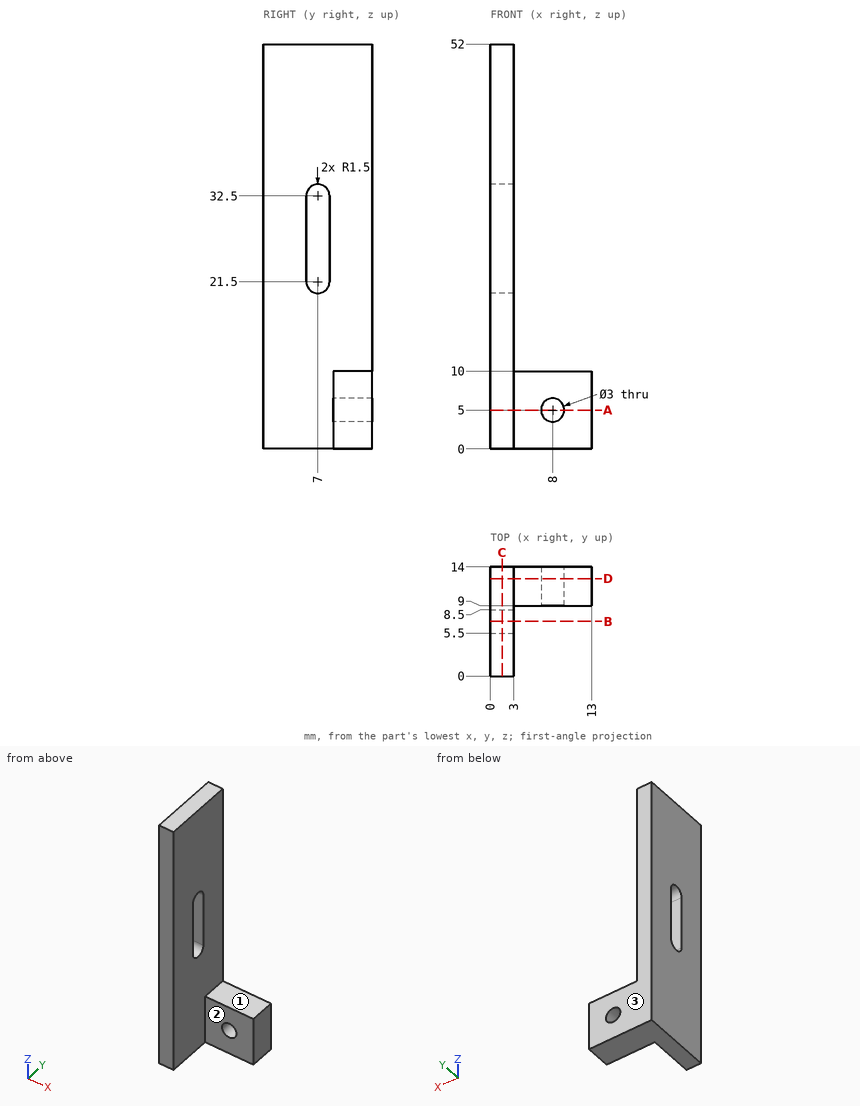
Job drawing, mm, ordinate dimensions from the low corner. One solid piece. Give positions to 0.01 mm unless a question says otherwise; leave off trailing zeros. Loops run counter-clockwise (first coordinate to the right, second up) from the corner with the lowest first, then second, coordinate; pieces in that order, holes last. Notation, with made-up numbers: M -30,-34.75 L -13,-34.75 A20 ccw -13,-15.75 Z; hole C -23.75,-3 d7. An arc over 180 degrees is marked long. Return JSON: item names as keys, results as strings.
1) Saw through at D-D, the plane y = 12.5. List the corners of the cut face in (x, z).
Calculated:
{"outline": "M 0,0 L 13,0 L 13,10 L 3,10 L 3,52 L 0,52 Z; hole C 8,5 d3"}
2) Drill centre lines: line 1 (Y direction, x = 1, z = 31); line 2 (Z direction, x = 8, y = 11.6); line 3 (Z direction, x = 3.25, y = 9.25). Where is each one in solid material? Low to high.
Calculated:
{"line 1": "y = 0 to 5.5, 8.5 to 14", "line 2": "z = 0 to 3.5, 6.5 to 10", "line 3": "z = 0 to 10"}
3) Saw through at B-B, the plane y = 7. List the corners of the cut face in (x, z), then the cut area to 3 significant figures.
Calculated:
{"outline": "M 0,0 L 3,0 L 3,20 L 0,20 Z; M 0,34 L 3,34 L 3,52 L 0,52 Z", "area": "114 mm2"}
4) Pull direction Y, two halves, no side cores. Call the marked faces 1, 2 and 3: released by +Y, released by -Y, zero draft, split by the parting line, or undercut.
Calculated:
{"face 1": "zero draft", "face 2": "released by -Y", "face 3": "released by +Y"}
5) Saw through at C-C, the plane x = 1.5. List the corners of the cut face in (y, z), then the cut area to 3 significant figures.
Calculated:
{"outline": "M 0,0 L 14,0 L 14,52 L 0,52 Z; hole M 5.5,21.5 A1.5 ccw 8.5,21.5 L 8.5,32.5 A1.5 ccw 5.5,32.5 Z", "area": "688 mm2"}
6) Saw through at A-A, the plane z = 5. List the corners of the cut face in (x, y).
Calculated:
{"outline": "M 0,0 L 3,0 L 3,9 L 6.5,9 L 6.5,14 L 0,14 Z; M 9.5,9 L 13,9 L 13,14 L 9.5,14 Z"}
7) Flat gauge pins, fed straight in: pin 1 Ø6 at (y, z) = (5, 11.5) entering from -X; pin 2 Ø2 at (y, z) = (10.5, 19) entering from +X; pin 3 Ø5.5 at (x, y) = (10.5, 11.5) entering from +Z. Where does each tip first touch, or does it go through?
Calculated:
{"pin 1": "stops at x = 0", "pin 2": "stops at x = 3", "pin 3": "stops at z = 10"}
